```python
from build123d import *

# Parameters (mm, degrees)
SKETCH1_R           = 30
SKETCH1_R_2         = 25
BOSS_EXTRUDE1_DEPTH = 5
BOSS_EXTRUDE2_START = -5
SKETCH2_R           = 2.55
BOSS_EXTRUDE2_DEPTH = 5
CIRPATTERN1_COUNT   = 3
FILLET1_R           = 1.5


with BuildPart() as part:
    # Sketch1 → Boss-Extrude1 (new body)
    with BuildSketch(Plane(origin=(0, 0, 0), x_dir=(1, 0, 0), z_dir=(0, 1, 0))):
        with Locations(Location((0, 0, 0), (0, 0, 270))):
            Circle(SKETCH1_R)
        with Locations(Location((0, 0, 0), (0, 0, 270))):
            Circle(SKETCH1_R_2, mode=Mode.SUBTRACT)
    extrude(amount=BOSS_EXTRUDE1_DEPTH)

    # Sketch2 → Boss-Extrude2 (add)
    with BuildSketch(Plane(origin=(0, 5, 0), x_dir=(1, 0, 0), z_dir=(0, 1, 0)).offset(BOSS_EXTRUDE2_START)):
        with BuildLine():
            Line((-4.75, 15.25), (-4.75, 24.544602258))
            ThreePointArc((-4.75, 24.544602258), (0, 25), (4.75, 24.544602258))
            Line((4.75, 24.544602258), (4.75, 15.25))
            ThreePointArc((4.75, 15.25), (0, 10.5), (-4.75, 15.25))
        make_face()
        with Locations(Location((0, 15.25, 0), (0, 0, 270))):
            Circle(SKETCH2_R, mode=Mode.SUBTRACT)
    boss_extrude2 = extrude(amount=BOSS_EXTRUDE2_DEPTH)

    # CirPattern1: Boss-Extrude2 ×3 about axis
    cirpattern1_axis = Axis((0, 0, 0), (0, 1, 0))
    for i in range(1, CIRPATTERN1_COUNT):
        add(boss_extrude2.rotate(cirpattern1_axis, i * 360 / CIRPATTERN1_COUNT))

    # Fillet1
    fillet1_edges = [part.edges().sort_by_distance(p)[0] for p in [
        (4.75, 2.5, -24.544602258),
        (-4.75, 2.5, -24.544602258),
        (18.881249081, 2.5, 16.385921797),
        (23.631249081, 2.5, 8.158680461),
        (-23.631249081, 2.5, 8.158680461),
        (-18.881249081, 2.5, 16.385921797),
    ]]
    fillet(fillet1_edges, radius=FILLET1_R)


solid = part.part
```
CAD build for the part. Positions are in the model's coordinates, mm. A direction names the side the tool comes from. Coordinates: 2 decimals unless noted, no trailing zeros. Write each loop counter-clockwise with the first axis right and the second up, starting at its lowest first coordinate (ties: lowest second). Pieces come first, ordered by that corner, then holes. Notation, with made-up numbers: (68.5, -3.5) -> (123.5, -3.5) arc R7 cw to (123.5, 4.5) -> close; hole circle Ø6 at (46, -35.75). An arc over 180 degrees is marked (long way). Return JSON: item names as keys, results as strings. Group by question number.
Q1. Drill centre lines: line 1 (Z direction, x = 11, y = 1.4); line 2 (X direction, y = 2.8, z = -19.5); line 3 (X direction, y = 3.2, z = -16.5). Where is each one in solid material? Low to high.
Q2. Cut at B-B, the plane x = 1.5. Give the cut face in (y, z), then the cut area to 3 significant figures.
Q3. Cut at A-A, the plane z = 0. Give the cut face in (x, y).
Q4. Cut at D-D, the plane y = 3.55. Give the cut face in (x, z) (3 decimals).
Q5. Which spindle directions (+Z, -Z, +X, -X, +Y, -Y) get a long thin tool onto all of the face, cutting with end or side? Do faces 1 (the face through (-23.34, 2.54, 7.29)), 2 (the face through (9, 0, 7)). Say none if no direction does.
Q6. Flat gauge pins, fed straight in: pin 1 (2 mm diameter, centred on x = -12, z = 21, fed in from +Y); pin 2 (1.5 mm diameter, centred on y = 3, z = -18, fed in from -X); pin 3 (2 mm diameter, centred on y = 2, z = -13, fed in from -X); pin 4 (3 mm diameter, centred on y = 2.5, z = -22.5, fed in from -X). Where does each tip first touch, or does it go through?
Q7. Cut at C-C, the plane z = -17. Give the cut face in (x, y), then the cut area to 3 significant figures.
Returned:
{
 "1": {"line 1": "z = -27.91 to -22.45, 3.42 to 6.35, 8.9 to 11.84, 22.45 to 27.91", "line 2": "x = -22.8 to -15.64, -4.75 to 4.75, 15.64 to 22.8", "line 3": "x = -25.05 to -18.78, -4.75 to -2.22, 2.22 to 4.75, 18.78 to 25.05"},
 "2": {"outline": "(0, -29.96) -> (5, -29.96) -> (5, -17.31) -> (0, -17.31) -> close; (0, -13.19) -> (5, -13.19) -> (5, -10.74) -> (0, -10.74) -> close; (0, 24.95) -> (5, 24.95) -> (5, 29.96) -> (0, 29.96) -> close", "area": "101 mm2"},
 "3": {"outline": "(-30, 0) -> (-25, 0) -> (-25, 5) -> (-30, 5) -> close; (25, 0) -> (30, 0) -> (30, 5) -> (25, 5) -> close"},
 "4": {"outline": "circle Ø60 at (0, 0); hole (-24.195, 6.292) arc R25 ccw to (-6.649, -24.1) arc R1.5 ccw to (-4.75, -22.654) -> (-4.75, -15.25) arc R4.75 cw to (4.75, -15.25) -> (4.75, -22.654) arc R1.5 ccw to (6.649, -24.1) arc R25 ccw to (24.195, 6.292) arc R1.5 ccw to (21.994, 7.213) -> (15.582, 3.511) arc R4.75 cw to (10.832, 11.739) -> (17.244, 15.44) arc R1.5 ccw to (17.546, 17.808) arc R25 ccw to (-17.546, 17.808) arc R1.5 ccw to (-17.244, 15.44) -> (-10.832, 11.739) arc R4.75 cw to (-15.582, 3.511) -> (-21.994, 7.213) arc R1.5 ccw to start; hole circle Ø5.1 at (-13.207, 7.625); hole circle Ø5.1 at (0, -15.25); hole circle Ø5.1 at (13.207, 7.625)"},
 "5": {"face 1": "+Y, -Y", "face 2": "+Z, -Z, +X, -X, -Y"},
 "6": {"pin 1": "stops at y = 5", "pin 2": "stops at x = -24.54", "pin 3": "stops at x = -27.5", "pin 4": "stops at x = -21.42"},
 "7": {"outline": "(-24.72, 0) -> (-18.33, 0) -> (-18.33, 5) -> (-24.72, 5) -> close; (-4.75, 0) -> (-1.85, 0) -> (-1.85, 5) -> (-4.75, 5) -> close; (1.85, 0) -> (4.75, 0) -> (4.75, 5) -> (1.85, 5) -> close; (18.33, 0) -> (24.72, 0) -> (24.72, 5) -> (18.33, 5) -> close", "area": "92.8 mm2"}
}
